Design review of the part built by this model. Coordinates are the model's own, in mm. A direction names the side the tool comes from. Coordinates: 2 decimals unless noted, no trailing zeros. Loops run counter-clockwise (first coordinate to the right, second up) from the corner with the lowest first, then second, coordinate; pieces in that order, holes last. Notation, with made-up numbers: (26, 21.25) -> (66, 21.25) arc R16 cw to (66, 33.25) -> close; hole circle Ø6 at (-22, 38). An arc over 180 degrees is marked (long way). Use a Markdown table: item, result. Add a question column.
Q1. Take a section at D-D on x = 25. Write out the cut boundary in (y, z).
Q2. For faces 4 (the face through (19, -96, 21)), 5 (the face through (11.772, -97.972, 19.265)), list the 3-axis set-ups (+Z, -Z, +X, -X, +Y, -Y) from which the entire face can be reached by the end or side of a thin tool; tool diameter is ignored.
Q3. Draft analysis for pull direction X (two halves, no side actions). For faces 1 (the face through (30, -98, 21)), 2 (the face through (23.61, -97.97, 38.06)), 3 (the face through (0, -49, 21)), state which applies: pulls with the +X half, pulls with the -X half, needs draft (parallel to the pull), parting line crosses it, or undercut.
Q4. Take a section at C-C on z = 21. Write out the cut boundary in (x, y).
Q5. For probe 1 along Z at (x, y) = (25, -98.6); probe 2 along X at (y, z) = (-97.9, 37); probe 3 along X at (y, z) = (-97, 21), list the stretches that pass through material, from the lowest coordinate up.
Q6. Take a section at B-B on x = 12. Write out the cut boundary in (y, z).
Q7. Clearance check with flat-ended pins moving along their axes: pin 1 Ø4 at (x, z) = (14, 25.5) entering from +Y; pin 2 Ø4 at (y, z) = (-89, 33) entering from +X. State where each tip first meets the part, or that it passes through.
Q8. Take a section at A-A on y = -21. Write out the cut boundary in (x, z), plus the area to 3 significant figures.
Autodesk Inventor part; units mm, degrees
ref_plane "YZ Plane" through (0, 0, 0) normal (1, 0, 0) x (0, 1, 0)
ref_plane "XZ Plane" through (0, 0, 0) normal (0, 1, 0) x (-1, 0, 0)
ref_plane "XY Plane" through (0, 0, 0) normal (0, 0, 1) x (1, 0, 0)
sketch "Sketch1" plane through (0, 0, 0) normal (0, 0, 1) x (1, 0, 0)
  point P0 (0, 0)
sketch "Sketch2" plane through (0, 0, 0) normal (0, 0, 1) x (1, 0, 0)
  line L0 (0, 0) -> (0, -100)
  line L1 (0, -100) -> (30, -100)
  line L2 (30, -100) -> (30, -96)
  line L3 (30, -96) -> (4, -96)
  line L4 (4, -96) -> (4, 0)
  line L5 (4, 0) -> (0, 0)
  dimension "d0" = 100
  dimension "d1" = 30
  dimension "d2" = 4
  dimension "d3" = 26
extrude "Extrusion1" add sketch "Sketch2" along normal blind 42
sketch "Sketch4" plane through (4, -96, 0) normal (0, 1, 0) x (1, 0, 0)
  line L0 (-4, -42) -> (26, -42)
  line L1 (-4, 0) -> (26, 0)
  line L2 (26, 0) -> (26, -42)
  line L3 (26, -42) -> (-4, -42)
  line L4 (-4, -42) -> (-4, 0)
  circle A0 centre (21, -37) radius 1.75
  circle A1 centre (21, -5) radius 1.75
  circle A2 centre (8, -21) radius 1.75
  dimension "d11" = 3.5
  dimension "d12" = 3.5
  dimension "d13" = 3.5
  dimension "d14" = 5
  dimension "d15" = 5
  dimension "d16" = 5
  dimension "d17" = 5
  dimension "d18" = 12
  dimension "d19" = 21
extrude "Extrusion3" cut sketch "Sketch4" against normal blind 4 contours A0 | A1 | A2
fillet "Fillet1" radius 3 1 edges at (4, -96, 21)
sketch "Sketch5" plane through (4, 0, 42) normal (1, 0, 0) x (0, 0, -1)
  line L0 (42, 0) -> (0, 0)
  line L1 (42, -100) -> (0, -100)
  line L2 (42, 0) -> (0, 0)
  line L3 (0, 0) -> (0, -100)
  line L4 (0, -100) -> (42, -100)
  line L5 (42, -100) -> (42, 0)
  circle A0 centre (21, -21) radius 6.8
  dimension "d23" = 13.6
  dimension "d24" = 21
  dimension "d25" = 21
extrude "Extrusion4" cut sketch "Sketch5" against normal blind 4 contours A0
properties part number "Suporte Direito"
Answer list:
| question | item | result |
|---|---|---|
| 1 | outline | (-100, 0) -> (-96, 0) -> (-96, 3.25) -> (-100, 3.25) -> close; (-100, 6.75) -> (-96, 6.75) -> (-96, 35.25) -> (-100, 35.25) -> close; (-100, 38.75) -> (-96, 38.75) -> (-96, 42) -> (-100, 42) -> close |
| 2 | face 4 | +Z, -Z, +X, +Y |
| 2 | face 5 | +Y, -Y |
| 3 | face 1 | pulls with the +X half |
| 3 | face 2 | undercut |
| 3 | face 3 | pulls with the -X half |
| 4 | outline | (0, -100) -> (10.25, -100) -> (10.25, -96) -> (7, -96) arc R3 cw to (4, -93) -> (4, -27.8) -> (0, -27.8) -> close; (0, -14.2) -> (4, -14.2) -> (4, 0) -> (0, 0) -> close; (13.75, -100) -> (30, -100) -> (30, -96) -> (13.75, -96) -> close |
| 5 | probe 1 | 0 to 3.25, 6.75 to 35.25, 38.75 to 42 |
| 5 | probe 2 | 0 to 23.25, 26.75 to 30 |
| 5 | probe 3 | 0 to 10.25, 13.75 to 30 |
| 6 | outline | (-100, 0) -> (-96, 0) -> (-96, 19.25) -> (-100, 19.25) -> close; (-100, 22.75) -> (-96, 22.75) -> (-96, 42) -> (-100, 42) -> close |
| 7 | pin 1 | y = -96 |
| 7 | pin 2 | x = 4 |
| 8 | outline | (0, 0) -> (4, 0) -> (4, 14.2) -> (0, 14.2) -> close; (0, 27.8) -> (4, 27.8) -> (4, 42) -> (0, 42) -> close |
| 8 | area | 114 mm² |
